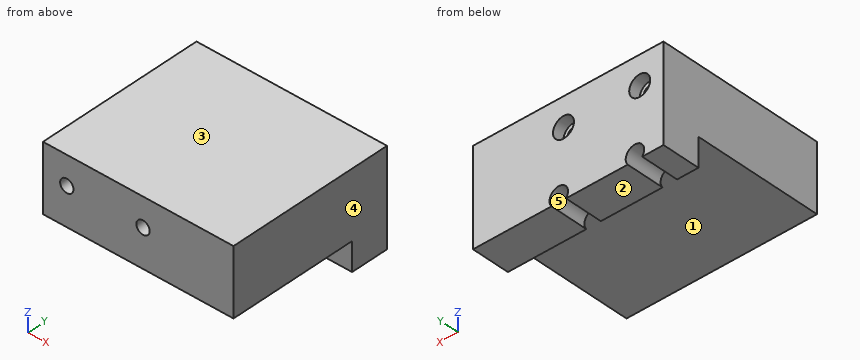
```python
from build123d import *

# Parameters (mm, degrees)
SKETCH_1_W                   = 100
SKETCH_1_H                   = 88
EXTRUDE_1_DEPTH              = 50
SKETCH_2_W                   = 15
SKETCH_2_H                   = 68
CUT_EXTRUDE_1_DEPTH          = 143.281411295
SKETCH_4_R                   = 4.85
CUT_EXTRUDE_3_DEPTH          = 143.281411295
HOLE_WIZARD_M6_1_D           = 7
HOLE_WIZARD_M6_1_CBORE_D     = 11
HOLE_WIZARD_M6_1_CBORE_DEPTH = 6


with BuildPart() as part:
    # 草图1 → 凸台-拉伸1 (new body)
    with BuildSketch(Plane.XY):
        with Locations((50, 44)):
            Rectangle(SKETCH_1_W, SKETCH_1_H)
    extrude(amount=EXTRUDE_1_DEPTH)

    # 草图2 → 切除-拉伸1 (cut, through all)
    with BuildSketch(Plane.ZY):
        with Locations((7.5, 34)):
            Rectangle(SKETCH_2_W, SKETCH_2_H)
    extrude(amount=-CUT_EXTRUDE_1_DEPTH, mode=Mode.SUBTRACT)

    # 草图4 → 切除-拉伸3 (cut, through all)
    with BuildSketch(Plane(origin=(0, 88, 0), x_dir=(1, 0, 0), z_dir=(0, 1, 0))):
        with Locations((15, -3)):
            Circle(SKETCH_4_R)
        with Locations((55, -3)):
            Circle(SKETCH_4_R)
    extrude(amount=-CUT_EXTRUDE_3_DEPTH, mode=Mode.SUBTRACT)

    # M6 六角凹头螺钉的柱形沉头孔1 (through all)
    with Locations(Plane(origin=(0, 88, 0), x_dir=(-1, 0, 0), z_dir=(0, 1, 0))):
        with Locations((-12.5, 35), (-52.5, 35)):
            CounterBoreHole(HOLE_WIZARD_M6_1_D / 2, HOLE_WIZARD_M6_1_CBORE_D / 2, HOLE_WIZARD_M6_1_CBORE_DEPTH)


solid = part.part
```
Model file for the job. Use its own axes, mm. Face numbers are marked on the shaded views. A direction names the side the tool comes from. Coordinates: 2 decimals unless noted, no trailing zeros. Order: outer loops, then holes, each group sorted by start corner. A loop starts at its lowest first (then second) coordinate and runs counter-clockwise, first axis right, second up. Notation, with made-up numbers: (85, -14.5) -> (92, -14.5) arc R16 cw to (92, 3.5) -> close; hole circle Ø2 at (4.25, 73). An arc over 180 degrees is marked (long way). Answer as a JSON object with one key per item and string values. Group by question number.
1) Cut at A-A, the plane z = 35. Write the cut outline in (x, y), then the cut area to 3 significant figures.
2) Cut at D-D, the plane z = 3. Write the cut outline in (x, y), then the cut area to 3 significant figures.
3) Pull direction Z, two halves, no side cores. Call the marked faces 3, 4 and 5: +Z half, -Z half, draft (parallel to the pull), parting line (faces both ways), or undercut.
4) Cut at C-C, the plane x = 12.5. Write the cut outline in (y, z), then the cut area to 3 significant figures.
5) Cut at B-B, the plane y = 73. Write the cut outline in (x, z).
6) Flat gauge pins, fed straight in: pin 1 (3 mm diameter, centred on x = 79.5, z = 10, fed in from -Y); pin 2 (8 mm diameter, centred on x = 12.5, z = 35, fed in from -Y); pin 3 (4 mm diameter, centred on x = 18, y = 56.5, fed in from -Z); pin 4 (8.5 mm diameter, centred on x = 15, z = 3, fed in from +Y). Where does each tip first touch, or does it go through?
7) Drill centre lines: L1, parallel to X at y = 76, z = 3; L2, parallel to X at y = 32.5, z = 33; L3, parallel to Z at x = 63.5, y = 6. Where is each one in solid material? Low to high.
8) Which spindle directions (+Z, -Z, +X, -X, +Y, -Y) get a long thin tool onto all of the face, cutting with end or side? Do the marked faces 1 and 2. Say none if no direction does.
Check values:
{
 "1": {"outline": "(0, 0) -> (9, 0) -> (9, 82) -> (7, 82) -> (7, 88) -> (0, 88) -> close; (16, 0) -> (49, 0) -> (49, 82) -> (47, 82) -> (47, 88) -> (18, 88) -> (18, 82) -> (16, 82) -> close; (56, 0) -> (100, 0) -> (100, 88) -> (58, 88) -> (58, 82) -> (56, 82) -> close", "area": "7,520 mm²"},
 "2": {"outline": "(0, 68) -> (10.15, 68) -> (10.15, 88) -> (0, 88) -> close; (19.85, 68) -> (50.15, 68) -> (50.15, 88) -> (19.85, 88) -> close; (59.85, 68) -> (100, 68) -> (100, 88) -> (59.85, 88) -> close", "area": "1,610 mm²"},
 "3": {"face 3": "+Z half", "face 4": "draft", "face 5": "undercut"},
 "4": {"outline": "(0, 15) -> (68, 15) -> (68, 7.16) -> (88, 7.16) -> (88, 29.5) -> (82, 29.5) -> (82, 31.5) -> (0, 31.5) -> close; (0, 38.5) -> (82, 38.5) -> (82, 40.5) -> (88, 40.5) -> (88, 50) -> (0, 50) -> close", "area": "2,600 mm²"},
 "5": {"outline": "(0, 0) -> (11.19, 0) arc R4.85 cw (long way) to (18.81, 0) -> (51.19, 0) arc R4.85 cw (long way) to (58.81, 0) -> (100, 0) -> (100, 50) -> (0, 50) -> close; hole circle Ø7 at (12.5, 35); hole circle Ø7 at (52.5, 35)"},
 "6": {"pin 1": "stops at y = 68", "pin 2": "stops at y = 0", "pin 3": "stops at z = 15", "pin 4": "passes through"},
 "7": {"L1": "x = 0 to 10.15, 19.85 to 50.15, 59.85 to 100", "L2": "x = 0 to 9.63, 15.37 to 49.63, 55.37 to 100", "L3": "z = 15 to 50"},
 "8": {"face 1": "-Z, +X, -X, -Y", "face 2": "-Z, +X, -X, +Y, -Y"}
}
